Here's how the part is built. I have some questions about the finished solid (model axes, mm). A direction names the side the tool comes from. Coordinates: 2 decimals unless noted, no trailing zeros. Write each loop counter-clockwise with the first axis right and the second up, starting at its lowest first coordinate (ties: lowest second). Pieces come first, ordered by that corner, then holes.
(1) For pin 1 Ø0.9 at (y, z) = (24, 2) entering from +X; pin 2 Ø1.5 at (y, z) = (15.5, 0.5) entering from -X, each with a flat end and sliding along its axis, tell me the tip position at first contact or that it passes through.
(2) Thinking about a two-plate mould opening in Y: for faces 1 (the flat face through (18, 35.878, 2)), 2 (the flat face through (26, 23, 0)), 3 (the flat face through (-2, 30, 2)), which applies, released by +Y, released by -Y, zero draft, split by the parting line, or undercut?
(3) Imagine slicing it at B-B, the plane z = 0.85. State how many separate pieces and enclosed holes the cut face has, plus the area to 3 significant figures.
(4) Which directions (+Z, -Z, +X, -X, +Y, -Y) give clear straight access to the entire face, cutting with the end or side of a thin tool? Please do faces 4 (the flat face through (45, 13, 2)), 5 (the cylindrical face through (15.376, 22.525, 1.521)), 6 (the flat face through (19.645, 4, 2)), 7 (the flat face through (-2, 9.999, 2)), 8 (the flat face through (16.61, 40, 2)).
(5) Imagine slicing it at D-D, the plane y = 31.5. List the corners of the cut face in (x, z) for me, plus the area to 3 significant figures.
(6) Imagine slicing it at C-C, the plane y = 17. List the corners of the cut face in (x, z) for me.
(7) Please list where these lines run through material, in increasing order: probe 1 along Y at (x, z) = (13, 1.25); probe 2 along X at (y, z) = (40.5, 0.35); probe 3 along Y at (x, z) = (43.5, 1.1).
(8) Imagine slicing it at A-A, the plane x = 30. List the corners of the cut face in (y, z) for me.
```python
from build123d import *

# Parameters (mm, degrees)
SKETCH_1_R          = 3.6
EXTRUDE_1_DEPTH     = 3
CUT_EXTRUDE_2_DEPTH = 1


with BuildPart() as part:
    # 草图1 → 凸台-拉伸1 (new body)
    with BuildSketch(Plane.XY.offset(3)):
        Polygon((46.131858504, 44.9999), (19.645182907, 44.9999), (19.645182907, 35.877980345), (16.61, 35.877980345), (16.61, 44.9999), (-3.867371496, 44.9999), (-3.867371496, 29.9998), (-0.867341496, 29.9998), (-0.867341496, 9.9991), (-3.867371496, 9.9991), (-3.867371496, 0), (16.61, 0), (16.61, 7.754820329), (19.645182907, 7.754820329), (19.645182907, 0), (46.131858504, 0), (46.131858504, 13.0005), (43.131858504, 13.0005), (43.131858504, 34.9994), (46.131858504, 34.9994), align=None)
        with Locations(Location((21.131658504, 22.4992, 0), (0, 0, 180))):
            Circle(SKETCH_1_R, mode=Mode.SUBTRACT)
        with BuildLine():
            Line((9.236684618, 23.64925), (14.226589495, 23.64925))
            ThreePointArc((14.226589495, 23.64925), (15.376589495, 22.49925), (14.226589495, 21.34925))
            Line((14.226589495, 21.34925), (9.236684618, 21.34925))
            ThreePointArc((9.236684618, 21.34925), (8.086684618, 22.49925), (9.236684618, 23.64925))
        make_face(mode=Mode.SUBTRACT)
        with BuildLine():
            Line((33.064389495, 21.33685), (28.074484618, 21.33685))
            ThreePointArc((28.074484618, 21.33685), (26.924484618, 22.48685), (28.074484618, 23.63685))
            Line((28.074484618, 23.63685), (33.064389495, 23.63685))
            ThreePointArc((33.064389495, 23.63685), (34.214389495, 22.48685), (33.064389495, 21.33685))
        make_face(mode=Mode.SUBTRACT)
    extrude(amount=-EXTRUDE_1_DEPTH)

    # 草图3 → 切除-拉伸2 (cut)
    with BuildSketch(Plane.XY.offset(3)):
        with BuildLine():
            Line((1.034005341, 39.645473757), (0.719902777, 39.645473757))
            add(Edge.make_bspline(
                [(0.719902777, 39.645473757), (0.72194993, 39.687144645), (0.725970484, 39.768985159), (0.744798774, 39.888309066), (0.771739651, 40.002363865), (0.809831105, 40.110233779), (0.857137383, 40.212872586), (0.91386741, 40.309872601), (0.98106126, 40.40086379), (1.057267995, 40.485002633), (1.140036634, 40.562190204), (1.229342573, 40.628845447), (1.3231876, 40.685163118), (1.421286999, 40.73224436), (1.524747563, 40.767584206), (1.632630421, 40.793805846), (1.745409557, 40.809582191), (1.822249579, 40.811277977), (1.861329059, 40.812140424)],
                knots=[0, 0, 0, 0, 1.10065271, 2.161652631, 3.183658789, 4.190468796, 5.17591951, 6.163126047, 7.15150782, 8.156236427, 9.156009102, 10.134482811, 11.092018607, 12.041330605, 13.001268258, 13.972401359, 14.968799086, 16, 16, 16, 16], degree=3))
            add(Edge.make_bspline(
                [(1.861329059, 40.812140424), (1.899707133, 40.811241967), (1.975118678, 40.809476532), (2.085180693, 40.794315503), (2.189957987, 40.770569912), (2.289245754, 40.737254495), (2.382251818, 40.692470068), (2.469674863, 40.638672529), (2.552555673, 40.576452698), (2.627162457, 40.503198884), (2.695670536, 40.4249965), (2.754772791, 40.341508596), (2.805385955, 40.255279311), (2.847573635, 40.165651109), (2.878629774, 40.071780081), (2.902207982, 39.975032878), (2.915535395, 39.874408067), (2.917580819, 39.806301511), (2.918620726, 39.77167568)],
                knots=[0, 0, 0, 0, 1.111607364, 2.184268762, 3.212621178, 4.221274766, 5.211760367, 6.196651075, 7.1921475, 8.207485113, 9.220403448, 10.201281604, 11.166441695, 12.114753415, 13.065576456, 14.026450734, 14.996634279, 16, 16, 16, 16], degree=3))
            add(Edge.make_bspline(
                [(2.918620726, 39.77167568), (2.916927463, 39.722927846), (2.913570652, 39.626287632), (2.884856275, 39.484272769), (2.840009764, 39.34667935), (2.786012407, 39.235942048), (2.731539963, 39.146708554), (2.682452456, 39.073239849), (2.624987645, 38.994134381), (2.558309147, 38.909657044), (2.483796274, 38.819146138), (2.400774111, 38.722656343), (2.308650629, 38.621184573), (2.243992128, 38.551878972), (2.210487713, 38.515966546)],
                knots=[0, 0, 0, 0, 1.184426356, 2.348067706, 3.509069118, 4.696110526, 5.333549288, 6.050745305, 6.844228056, 7.710549037, 8.667450064, 9.695053472, 10.805634456, 12, 12, 12, 12], degree=3))
            Line((2.210487713, 38.515966546), (1.334786591, 37.581371193))
            Line((1.334786591, 37.581371193), (2.963492521, 37.581371193))
            Line((2.963492521, 37.581371193), (2.963492521, 37.222396834))
            Line((2.963492521, 37.222396834), (0.585287393, 37.222396834))
            Line((0.585287393, 37.222396834), (1.942659188, 38.670914462))
            add(Edge.make_bspline(
                [(1.942659188, 38.670914462), (1.975707074, 38.705412769), (2.039185301, 38.771676955), (2.128967878, 38.868419915), (2.209606867, 38.958169456), (2.281624259, 39.040756005), (2.343457765, 39.117387572), (2.398329997, 39.185582276), (2.442295588, 39.248336726), (2.490010983, 39.32107734), (2.536224965, 39.409889657), (2.575937321, 39.518423347), (2.600152169, 39.630150599), (2.603057005, 39.705652636), (2.604518162, 39.743630808)],
                knots=[0, 0, 0, 0, 1.329631726, 2.553950428, 3.673215718, 4.687767853, 5.603093632, 6.413772471, 7.123043292, 7.734684054, 8.834405432, 9.900288307, 10.943827018, 12, 12, 12, 12], degree=3))
            add(Edge.make_bspline(
                [(2.604518162, 39.743630808), (2.60388242, 39.767512207), (2.602629494, 39.814577857), (2.591571796, 39.883583616), (2.57486129, 39.95014843), (2.550916032, 40.014477049), (2.519309292, 40.075922701), (2.480835912, 40.134560181), (2.436445849, 40.191249147), (2.385094579, 40.244402445), (2.328683059, 40.29308365), (2.26908881, 40.336207736), (2.206038706, 40.372246846), (2.139798583, 40.401790343), (2.070553114, 40.424965725), (1.998168369, 40.441024304), (1.922844353, 40.451106788), (1.871410857, 40.45247096), (1.845203258, 40.453166065)],
                knots=[0, 0, 0, 0, 0.991446411, 1.95395049, 2.89581595, 3.838931463, 4.798493298, 5.75982156, 6.748411868, 7.785213223, 8.824556874, 9.840280684, 10.836137867, 11.835679398, 12.848801643, 13.863922112, 14.911575587, 16, 16, 16, 16], degree=3))
            add(Edge.make_bspline(
                [(1.845203258, 40.453166065), (1.817832425, 40.452451033), (1.764080629, 40.451046827), (1.685161596, 40.441224163), (1.609875819, 40.424278323), (1.538033916, 40.401101648), (1.46951433, 40.3716431), (1.404650286, 40.334951355), (1.343587397, 40.291167862), (1.286210873, 40.241527305), (1.233346894, 40.186259704), (1.186900018, 40.124649741), (1.146316004, 40.057822326), (1.110906771, 39.985957775), (1.082151081, 39.908403995), (1.06017793, 39.82543629), (1.042791083, 39.737414909), (1.036982563, 39.676629824), (1.034005341, 39.645473757)],
                knots=[0, 0, 0, 0, 1.031018746, 2.02475058, 2.990194455, 3.934040569, 4.864654155, 5.795059489, 6.735614925, 7.690564532, 8.649604399, 9.611025574, 10.590972636, 11.591080095, 12.624614302, 13.701020113, 14.821632451, 16, 16, 16, 16], degree=3))
        make_face()
    extrude(amount=-CUT_EXTRUDE_2_DEPTH, mode=Mode.SUBTRACT)


solid = part.part
```
Recorded:
1. pin 1: stops at x = 43.13
1. pin 2: stops at x = -0.87
2. face 1: released by +Y
2. face 2: zero draft
2. face 3: undercut
3. separate pieces: 1
3. enclosed holes: 3
3. area: 2,000 mm2
4. face 4: +Z, -Z, +X
4. face 5: +Z, -Z
4. face 6: +Z, -Z, -Y
4. face 7: +Z, -Z, -X
4. face 8: +Z, -Z, +Y
5. outline: (-3.87, 0) - (43.13, 0) - (43.13, 3) - (-3.87, 3) - close
5. area: 141 mm2
6. outline: (-0.87, 0) - (43.13, 0) - (43.13, 3) - (-0.87, 3) - close
7. probe 1: y = 0 to 21.35, 23.65 to 45
7. probe 2: x = -3.87 to 16.61, 19.65 to 46.13
7. probe 3: y = 0 to 13, 35 to 45
8. outline: (0, 0) - (21.34, 0) - (21.34, 3) - (0, 3) - close; (23.64, 0) - (45, 0) - (45, 3) - (23.64, 3) - close
